For this review, take the finished solid that the model builds, in its own axes (mm). A direction names the side the tool comes from. Coordinates: 2 decimals unless noted, no trailing zeros. Loops run counter-clockwise (first coordinate to the right, second up) from the corner with the lowest first, then second, coordinate; pieces in that order, holes last. Notation, with made-up numbers: (79, 84.25) -> (99, 84.25) arc R31 cw to (99, 109.25) -> close; hole circle Ø8 at (-2, 44.5). An arc over 180 degrees is marked (long way). Use a Markdown table: item, result.
from build123d import *

# Parameters (mm, degrees)
F1_DEPTH = 220


# Not quite as in the source:
# - the program builds the solid bodies; features that only make, move or delete a surface that nothing else refers to are left out


with BuildPart() as f1:
    # F0 (on Front) → F1 (new body)
    with BuildSketch(Plane.XZ):
        with BuildLine():
            Line((-178.3572353468, 80.260755906), (-178.3572353468, -80.260755906))
            Line((-178.3572353468, -80.260755906), (-138.3572353468, -80.260755906))
            Line((-138.3572353468, -80.260755906), (-138.3572353468, -110.260755906))
            Line((-138.3572353468, -110.260755906), (-118.3572353468, -110.260755906))
            Line((-118.3572353468, -110.260755906), (-118.3572353468, -80.260755906))
            Line((-118.3572353468, -80.260755906), (118.3572353468, -80.260755906))
            Line((118.3572353468, -80.260755906), (118.3572353468, -110.260755906))
            Line((118.3572353468, -110.260755906), (138.3572353468, -110.260755906))
            Line((138.3572353468, -110.260755906), (138.3572353468, -80.260755906))
            Line((138.3572353468, -80.260755906), (178.3572353468, -80.260755906))
            Line((178.3572353468, -80.260755906), (178.3572353468, 80.260755906))
            Line((178.3572353468, 80.260755906), (148.9576588225, 80.260755906))
            ThreePointArc((148.9576588225, 80.260755906), (0, 0), (-148.9576588225, 80.260755906))
            Line((-148.9576588225, 80.260755906), (-178.3572353468, 80.260755906))
        make_face()
    extrude(amount=F1_DEPTH)


solid = f1.part
(1) Take a section at D-D on x = 25.5. Write out the cut boundary in (y, z), plus the area to 3 significant figures.
Found:
| item | result |
|---|---|
| outline | (-220, -80.26) -> (0, -80.26) -> (0, 1.83) -> (-220, 1.83) -> close |
| area | 18,100 mm^2 |
(2) For pin 1 Ø2 at (x, y) = (99, -106) entering from +Z; pin 2 Ø2 at (x, y) = (-65, -127.5) entering from +Z; pin 3 Ø12 at (x, y) = (-153, -96.5) entering from -Z, all flat-tipped, find the tip position at first contact; note any pin that passes through.
Found:
| item | result |
|---|---|
| pin 1 | stops at z = 30.67 |
| pin 2 | stops at z = 12.66 |
| pin 3 | stops at z = -80.26 |
(3) Take a section at B-B on y = -152. Write out the cut boundary in (x, z).
Found:
| item | result |
|---|---|
| outline | (-178.36, -80.26) -> (-138.36, -80.26) -> (-138.36, -110.26) -> (-118.36, -110.26) -> (-118.36, -80.26) -> (118.36, -80.26) -> (118.36, -110.26) -> (138.36, -110.26) -> (138.36, -80.26) -> (178.36, -80.26) -> (178.36, 80.26) -> (148.96, 80.26) arc R178.36 cw to (-148.96, 80.26) -> (-178.36, 80.26) -> close |
(4) Take a section at A-A on z = 65. Write out the cut boundary in (x, y), plus the area to 3 significant figures.
Found:
| item | result |
|---|---|
| outline | (-178.36, -220) -> (-137.7, -220) -> (-137.7, 0) -> (-178.36, 0) -> close; (137.7, -220) -> (178.36, -220) -> (178.36, 0) -> (137.7, 0) -> close |
| area | 17,900 mm^2 |
(5) Take a section at C-C on z = 31. Write out the cut boundary in (x, y), plus the area to 3 significant figures.
Found:
| item | result |
|---|---|
| outline | (-178.36, -220) -> (-100.48, -220) -> (-100.48, 0) -> (-178.36, 0) -> close; (100.48, -220) -> (178.36, -220) -> (178.36, 0) -> (100.48, 0) -> close |
| area | 34,300 mm^2 |
(6) Mouldability with a two-part tool opening along X and no side actions: class faces 1 (the face through (-2, -108, -80.261)), 2 (the face through (-178.357, -108, 1)), 3 (the face through (158, -108, -80.261)) as pulls with the +X half, pulls with the -X half, needs draft (parallel to the pull), parting line crosses it, or undercut.
Found:
| item | result |
|---|---|
| face 1 | undercut |
| face 2 | pulls with the -X half |
| face 3 | needs draft |
(7) For line 1 along Z through (x, y) = (149, -102.5); line 2 along X through (y, z) = (-103.5, -84.5); line 3 along X through (y, z) = (-132.5, 62), list the stretches that pass through material, from the lowest coordinate up.
Found:
| item | result |
|---|---|
| line 1 | z = -80.26 to 80.26 |
| line 2 | x = -138.36 to -118.36, 118.36 to 138.36 |
| line 3 | x = -178.36 to -135.18, 135.18 to 178.36 |
(8) For faces 4 (the face through (-118.357, -108, -95)), 5 (the face through (138.357, -108, -95)), 6 (the face through (-159, -108, -80.261)), 7 (the face through (178.357, -108, -1)), list the 3-axis set-ups (+Z, -Z, +X, -X, +Y, -Y) from which the entire face can be reached by the end or side of a thin tool; tool diameter is ignored.
Found:
| item | result |
|---|---|
| face 4 | -Z, +Y, -Y |
| face 5 | -Z, +X, +Y, -Y |
| face 6 | -Z, -X, +Y, -Y |
| face 7 | +Z, -Z, +X, +Y, -Y |
